from build123d import *

# Parameters (mm, degrees)
PAD_DEPTH       = 6
POCKET_DEPTH    = 3
FILLET_R        = 1
CHAMFER_SIZE    = 2
SKETCH002_R     = 1.65
POCKET001_DEPTH = 6.001
POCKET002_DEPTH = 2.5


with BuildPart() as part:
    # Sketch → Pad (new body)
    with BuildSketch(Plane.XY):
        with BuildLine():
            Line((5.733466, 35.070521), (5.733466, 26))
            ThreePointArc((3.733466, 24), (5.14768, 24.585786), (5.733466, 26))
            Line((3.733466, 24), (-24.565653, 24))
            ThreePointArc((-26.565653, 26), (-25.979867, 24.585786), (-24.565653, 24))
            Line((-26.565653, 26), (-26.565653, 35))
            ThreePointArc((-26.565653, 35), (-27.15144, 36.414214), (-28.565653, 37))
            Line((-36.2, 37), (-28.565653, 37))
            ThreePointArc((-36.2, 37), (-37.614214, 36.414214), (-38.2, 35))
            Line((-38.2, 35), (-38.2, 2))
            ThreePointArc((-38.2, 2), (-37.614214, 0.585786), (-36.2, 0))
            Line((-25.8, 0), (-36.2, 0))
            Line((-25.8, 0), (-24.418427, 0))
            ThreePointArc((-24.418427, 0), (-23.841077, 0.183503), (-23.475618, 0.666667))
            ThreePointArc((-19.704382, 0.666667), (-21.59, 2), (-23.475618, 0.666667))
            ThreePointArc((-19.704382, 0.666667), (-19.338923, 0.183503), (-18.761573, 0))
            Line((-18.761573, 0), (-14.258427, 0))
            ThreePointArc((-14.258427, 0), (-13.681077, 0.183503), (-13.315618, 0.666667))
            ThreePointArc((-9.544382, 0.666667), (-11.43, 2), (-13.315618, 0.666667))
            ThreePointArc((-9.544382, 0.666667), (-9.178923, 0.183503), (-8.601573, 0))
            Line((-8.601573, 0), (-2.828427, 0))
            ThreePointArc((-2.828427, 0), (-2.251077, 0.183503), (-1.885618, 0.666667))
            ThreePointArc((1.885618, 0.666667), (0, 2), (-1.885618, 0.666667))
            ThreePointArc((1.885618, 0.666667), (2.251077, 0.183503), (2.828427, 0))
            Line((2.828427, 0), (8.601573, 0))
            ThreePointArc((8.601573, 0), (9.178923, 0.183503), (9.544382, 0.666667))
            ThreePointArc((13.315618, 0.666667), (11.43, 2), (9.544382, 0.666667))
            ThreePointArc((13.315618, 0.666667), (13.681077, 0.183503), (14.258427, 0))
            Line((14.258427, 0), (18.761573, 0))
            ThreePointArc((18.761573, 0), (19.338923, 0.183503), (19.704382, 0.666667))
            ThreePointArc((23.475618, 0.666667), (21.59, 2), (19.704382, 0.666667))
            ThreePointArc((23.475618, 0.666667), (23.841077, 0.183503), (24.418427, 0))
            Line((24.418427, 0), (25.8, 0))
            Line((25.8, 0), (35.8, 0))
            ThreePointArc((35.8, 0), (37.214214, 0.585786), (37.8, 2))
            Line((37.8, 35), (37.8, 2))
            ThreePointArc((37.8, 35), (37.214214, 36.414214), (35.8, 37))
            Line((8.25988, 37), (35.8, 37))
            ThreePointArc((8.25988, 37), (6.519553, 36.659991), (5.733466, 35.070521))
        make_face()
        Polygon((7.071068, 13.5), (0, 20.571068), (-7.071068, 13.5), (0, 6.428932), align=None, mode=Mode.SUBTRACT)
    extrude(amount=PAD_DEPTH)

    # Sketch001 (on Face40 of Pad) → Pocket (cut)
    with BuildSketch(Plane.XY.offset(6)):
        with BuildLine():
            Line((-26.565653, 34), (25.8, 34))
            ThreePointArc((27.8, 32), (27.214214, 33.414214), (25.8, 34))
            Line((27.8, 32), (27.8, -3.158395))
            Line((27.8, -3.158395), (-26.565653, -3.158395))
            Line((-26.565653, -3.158395), (-26.565653, 34))
        make_face()
    extrude(amount=-POCKET_DEPTH, mode=Mode.SUBTRACT)

    # Fillet
    fillet_edges = [part.edges().sort_by_distance(p)[0] for p in [
        (-26.565653, 0, 4.5),
        (27.8, 0, 4.5),
        (5.733466, 34, 4.5),
    ]]
    fillet(fillet_edges, radius=FILLET_R)

    # Chamfer
    chamfer_edges = [part.edges().sort_by_distance(p)[0] for p in [
        (3.535534, 9.964466, 0),
        (3.535534, 17.035534, 0),
        (-3.535534, 17.035534, 0),
        (-3.535534, 9.964466, 0),
    ]]
    chamfer(chamfer_edges, length=CHAMFER_SIZE)

    # Sketch002 (on Face49 of Chamfer) → Pocket001 (cut, through all)
    with BuildSketch(Plane.XY.offset(6)):
        with Locations((-32.57, 18.5)):
            Circle(SKETCH002_R)
        with Locations((32.8, 18.5)):
            Circle(SKETCH002_R)
    extrude(amount=-POCKET001_DEPTH, mode=Mode.SUBTRACT)

    # Sketch003 (on Face1 of Pocket001) → Pocket002 (cut)
    with BuildSketch(Plane(origin=(0, 0, 0), x_dir=(1, 0, 0), z_dir=(0, 0, -1))):
        Polygon((-29.928623, -20.025), (-29.928623, -16.975), (-32.57, -15.45), (-35.211377, -16.975), (-35.211377, -20.025), (-32.57, -21.55), align=None)
        Polygon((35.441377, -20.025), (35.441377, -16.975), (32.8, -15.45), (30.158623, -16.975), (30.158623, -20.025), (32.8, -21.55), align=None)
    extrude(amount=-POCKET002_DEPTH, mode=Mode.SUBTRACT)


solid = part.part
Input: part model. Units: mm. Frame: model coordinates. A direction names the side the tool comes from. Round coordinates to 2 decimals unless told otherwise and drop trailing zeros. Order: outer loops, then holes, each group sorted by start corner. A loop starts at its lowest first (then second) coordinate and runs counter-clockwise, first axis right, second up.
1. Cut plane D-D, the plane x = 17. Output: boundary loops of the cut face in (y, z), then the cut area to 3 significant figures.
The answers:
outline: (0, 0) - (37, 0) - (37, 6) - (34, 6) - (34, 3) - (0, 3) - close
area: 120 mm2
2. Cut plane A-A, the plane z = 3.75. Output: boundary loops of the cut face in (x, y), then the cut area to 3 significant figures.
The answers:
outline: (-38.2, 2) arc R2 ccw to (-36.2, 0) - (-27.57, 0) arc R1 ccw to (-26.57, 1) - (-26.57, 35) arc R2 ccw to (-28.57, 37) - (-36.2, 37) arc R2 ccw to (-38.2, 35) - close; (5.73, 35) arc R1 ccw to (6.73, 34) - (25.8, 34) arc R2 cw to (27.8, 32) - (27.8, 1) arc R1 ccw to (28.8, 0) - (35.8, 0) arc R2 ccw to (37.8, 2) - (37.8, 35) arc R2 ccw to (35.8, 37) - (8.26, 37) arc R2 ccw to (5.73, 35.07) - close; hole circle Ø3.3 at (-32.57, 18.5); hole circle Ø3.3 at (32.8, 18.5)
area: 845 mm2
3. Mould query, pull axis Y, two halves, no side actions, for faces 5 (the face through (-35.211, 18, 1)), 6 (the face through (31, 0, 2)), 7 (the face through (-27.14, 36.4, 2.96)). Classes: released by +Y, released by -Y, zero draft, split by the parting line, or undercut.
The answers:
face 5: undercut
face 6: released by -Y
face 7: released by +Y
4. Pin query (flat end, axial travel): P1, Ø3, axis at x = -34, z = 3.5, coming from the +Y side; P2, Ø2.5, axis at x = -9, z = 1, coming from the +Y side; P3, Ø5, axis at x = 15, y = 15.5, coming from the +Z side; P4, Ø2.5, axis at x = 32.8, y = 18.5, coming from the +Z side. Return the tip coordinate at first contact, or that it passes through.
The answers:
P1: stops at y = 37
P2: stops at y = 24
P3: stops at z = 3
P4: passes through
5. Cut plane B-B, the plane x = -4.5. Output: boundary loops of the cut face in (y, z), then the cut area to 3 significant figures.
The answers:
outline: (0, 0) - (8.1, 0) - (10.93, 2) - (10.93, 3) - (0, 3) - close; (16.07, 2) - (18.9, 0) - (24, 0) - (24, 3) - (16.07, 3) - close
area: 50.9 mm2
6. Cut plane C-C, the plane y = 18.5. State how many separate pieces and enclosed holes the cut face has, then the cut area to 3 significant figures.
The answers:
separate pieces: 4
enclosed holes: 0
area: 225 mm2
7. Set-up query: faces 1 (the face through (3.486, 9.915, 2.493)), 2 (the face through (31.5, 20.8, 1.2)), 3 (the face through (27.8, 17, 5)), 4 (the face through (-10, 24, 1)). Return all of +Z, -Z, +X, -X, +Y, -Y with unobstructed straight access to the full face (end or side cutting, diameter ignored); none if empty.
The answers:
face 1: +Z, -Z
face 2: -Z
face 3: +Z, -Y
face 4: +Z, -Z, +Y
8. Material intervals for line 1 (X direction, y = 8, z = 3.5); line 2 (Y direction, x = 32.8, z = 4.7); line 3 (X direction, y = 32, z = 2), sorted ascending.
The answers:
line 1: x = -38.2 to -26.57, 27.8 to 37.8
line 2: y = 0 to 16.85, 20.15 to 37
line 3: x = -38.2 to -26.57, 5.73 to 37.8
